For this review, use the dimensioned drawing (mm, ordinates from the lowest corner) and the shaded views. A direction names the side the tool comes from. Coordinates: 2 decimals unless noted, no trailing zeros. Loops run counter-clockwise (first coordinate to the right, second up) from the corner with the lowest first, then second, coordinate; pieces in that order, holes last. Notation, with made-up numbers: M 5.5,82.25 L 13.5,82.25 A9 ccw 13.5,96.25 Z; hole C 41.5,88.25 d3. An arc over 180 degrees is marked long. Write item = value, one per line.
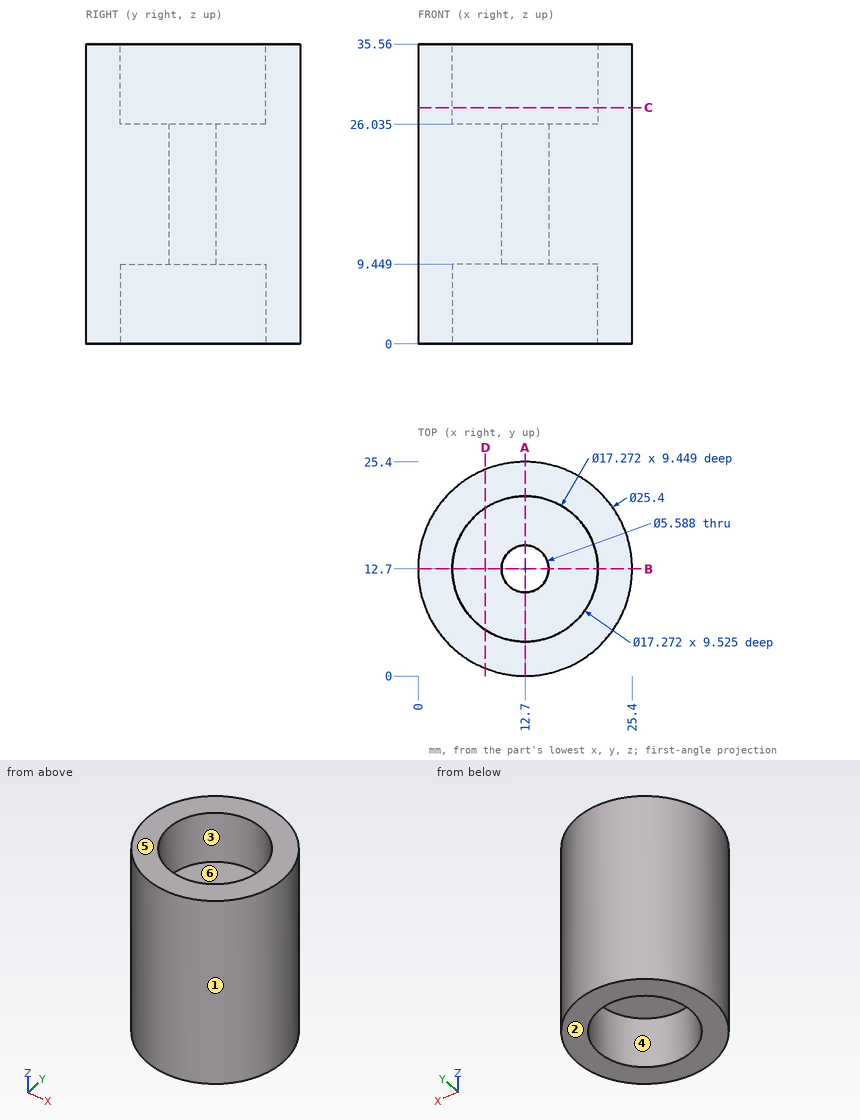
Q1. Add section A-A (x = 12.7). Write out the cut boundary in (y, z) (1 decimal).
Solved:
outline = M 0,0 L 4.1,0 L 4.1,9.4 L 9.9,9.4 L 9.9,26 L 4.1,26 L 4.1,35.6 L 0,35.6 Z; M 15.5,9.4 L 21.3,9.4 L 21.3,0 L 25.4,0 L 25.4,35.6 L 21.3,35.6 L 21.3,26 L 15.5,26 Z
Q2. Add section D-D (x = 8). Write out the cut boundary in (y, z) (1 decimal), and give its area (3 significant figures).
Solved:
outline = M 0.9,0 L 5.5,0 L 5.5,9.4 L 19.9,9.4 L 19.9,0 L 24.5,0 L 24.5,35.6 L 19.9,35.6 L 19.9,26 L 5.5,26 L 5.5,35.6 L 0.9,35.6 Z
area = 564 mm²
Q3. Draft analysis for pull direction X (two halves, no side actions). For the marked faces 1, 2 and 3, state which applies: +X half, -X half, draft (parallel to the pull), parting line (faces both ways), or undercut.
Solved:
face_1 = parting line
face_2 = draft
face_3 = undercut
Q4. For pin 1 Ø2 at (x, z) = (20, 13.5) entering from +Y; pin 2 Ø1 at (y, z) = (8.5, 18) entering from -X; pin 3 Ø6 at (x, y) = (15, 16) entering from -Z, all flat-tipped, find the tip position at first contact; note any pin that passes through.
Solved:
pin_1 = 23.73
pin_2 = 0.55
pin_3 = 9.45
Q5. For line 1 along Y through (x, z) = (12.7, 31.5); line 2 along Y through (x, z) = (12.7, 13.5); line 3 along Z through (x, y) = (8.5, 19.25) (1 decimal), list the stretches that pass through material, from the lowest coordinate up.
Solved:
line_1 = 0 to 4.06, 21.34 to 25.4
line_2 = 0 to 9.91, 15.49 to 25.4
line_3 = 9.4 to 26
Q6. Machinability: for the marked faces 4, 5 and 6, which of the approach directions +Z, -Z, +X, -X, +Y, -Y give a long, thin tool a straight path to every point of the face, cutting with its end or side? Answer none if there is none.
Solved:
face_4 = -Z
face_5 = +Z, +X, -X, +Y, -Y
face_6 = +Z
Q7. Add section C-C (z = 28). Write out the cut boundary in (x, y), and give its area (3 significant figures).
Solved:
outline = C 12.7,12.7 d25.4; hole C 12.7,12.7 d17.27
area = 272 mm²
